Here's how the part is built. I have some questions about the finished solid (model axes, mm). A direction names the side the tool comes from. Give positions to 0.01 mm unless a question says otherwise; leave off trailing zeros. Loops run counter-clockwise (first coordinate to the right, second up) from the corner with the lowest first, then second, coordinate; pieces in that order, holes last. Notation, with made-up numbers: (67, -14) - (110, -14) arc R28 ccw to (110, 19) - close; hole circle Ø4 at (8, 17). An arc over 180 degrees is marked (long way). Return JSON: item names as keys, results as strings. Group by question number.
(1) I need wall thicknesses on probe 1 along Y at (x, z) = (34.5, -22); probe 2 along X at (y, z) = (1, 29.5); probe 3 along X at (y, z) = (7, -34). Which ranges of each line are inside material? Lowest first, please. Write a range as [from, to].
(2) If we section it at A-A (x = 26): Please give me the cut outline in (y, z).
(3) If we mould it in two halves opening along Z, with no side actions, what happens to faces 1 (the flat face through (37, 7.493, 31)), 2 (the cylindrical face through (-92.62, -0.38, 51.75)), 3 (the flat face through (37.2, 6.2, -24.3)), 4 (the flat face through (37.2, 7.239, 27.5))? For each: released by +Z, released by -Z, zero draft, split by the parting line, or undercut.
(4) On a 3-axis mill with a long thin cutter (end or side, diameter ignored), from which of +Z, -Z, +X, -X, +Y, -Y can I reach the whole of each face in a straight line? I mean faces 5 (the flat face through (-19.051, 6.303, 34.262)), 6 (the flat face through (-81.539, 3, -2)), 7 (the flat face through (53, 3, -52.031)). Say none if no direction works.
(5) For P1, Ø3, axis at y = 4.5, z = 35, coming from the -X side; P2, Ø2, axis at x = -68, z = -18.5, coming from the +Y side; P3, Ø2, axis at x = -37.5, y = 4, coming from the -Z side; P4, Ø1.2, axis at y = 6.5, z = 26.5, coming from the -X side, each with a flat end and sliding along its axis, tell me the tip position at first contact or that it passes through.
(6) If we section it at C-C (x = -13): Please give me the cut outline in (y, z).
(7) If we section it at B-B (z = 2.5): Please give me the cut outline in (x, y).
```python
from build123d import *

# Parameters (mm, degrees)
F1_DEPTH   = 0.762
F2_W       = 166.2938
F2_H       = 100.7999
F3_DEPTH   = 5.08
F4_W       = 14.478
F4_H       = 7.874
F4_R       = 1.27
F4_W_2     = 7.874
F4_H_2     = 14.478
F5_DEPTH   = 2.413
F6_SIZE2   = 3.80999
F6_SIZE    = 2.41299
F6_2_SIZE2 = 3.80999
F6_2_SIZE  = 2.41299
F6_3_SIZE2 = 3.80999
F6_3_SIZE  = 2.41299
F6_4_SIZE2 = 3.80999
F6_4_SIZE  = 2.41299
F6_5_SIZE2 = 3.80999
F6_5_SIZE  = 2.41299
F6_6_SIZE2 = 3.80999
F6_6_SIZE  = 2.41299
F6_7_SIZE2 = 3.80999
F6_7_SIZE  = 2.41299
F6_8_SIZE2 = 3.80999
F6_8_SIZE  = 2.41299
F6_9_SIZE2 = 3.80999
F6_9_SIZE  = 2.41299
F7_SIZE2   = 3.80999
F7_SIZE    = 2.41299
F7_2_SIZE2 = 3.80999
F7_2_SIZE  = 2.41299
F7_3_SIZE2 = 3.80999
F7_3_SIZE  = 2.41299
F7_4_SIZE2 = 3.80999
F7_4_SIZE  = 2.41299
F7_5_SIZE2 = 3.80999
F7_5_SIZE  = 2.41299
F7_6_SIZE2 = 3.80999
F7_6_SIZE  = 2.41299
F7_7_SIZE2 = 3.80999
F7_7_SIZE  = 2.41299
F9_DEPTH   = 73.533
F11_DEPTH  = 64.2493
F12_W      = 40.005
F12_H      = 5.08
F13_DEPTH  = 3.34264


# Not quite as in the source:
# - a fillet or chamfer is up to 0.001 mm smaller than in the source, because OpenCascade refuses the exact size


with BuildPart() as f1:
    # F0 (on Front) → F1 (new body)
    with BuildSketch(Plane.XZ):
        with BuildLine():
            ThreePointArc((96.43872, 42.67327), (92.7189761211, 51.6535261211), (83.73872, 55.37327))
            Line((83.73872, 55.37327), (-83.73872, 55.37327))
            ThreePointArc((-83.73872, 55.37327), (-92.7189761211, 51.6535261211), (-96.43872, 42.67327))
            Line((-96.43872, 42.67327), (-96.43872, -42.67327))
            ThreePointArc((-96.43872, -42.67327), (-92.7189761211, -51.6535261211), (-83.73872, -55.37327))
            Line((-83.73872, -55.37327), (83.73872, -55.37327))
            ThreePointArc((83.73872, -55.37327), (92.7189761211, -51.6535261211), (96.43872, -42.67327))
            Line((96.43872, -42.67327), (96.43872, 42.67327))
        make_face()
    extrude(amount=F1_DEPTH)

    # F2 (on face) → F3 (join)
    with BuildSketch(Plane(origin=(0, 0, 0), x_dir=(-1, 0, 0), z_dir=(0, 1, 0))):
        with Locations((-1.60782, -1.63068)):
            Rectangle(F2_W, F2_H)
    extrude(amount=F3_DEPTH)

    # F4 (on face) → F5 (join)
    with BuildSketch(Plane(origin=(0, 5.08, 0), x_dir=(-1, 0, 0), z_dir=(0, 1, 0))):
        with Locations((-63.98768, 33.78327)):
            Rectangle(F4_W, F4_H)
        with Locations((-63.98768, 33.78327)):
            Circle(F4_R, mode=Mode.SUBTRACT)
        with Locations((-63.98768, -31.87573)):
            Rectangle(F4_W, F4_H)
        with Locations((-63.98768, -31.87573)):
            Circle(F4_R, mode=Mode.SUBTRACT)
        with Locations((62.22492, 33.78327)):
            Rectangle(F4_W, F4_H)
        with Locations((62.22492, 33.78327)):
            Circle(F4_R, mode=Mode.SUBTRACT)
        with Locations((62.22492, -31.87573)):
            Rectangle(F4_W, F4_H)
        with Locations((62.22492, -31.87573)):
            Circle(F4_R, mode=Mode.SUBTRACT)
        with Locations((-37.26942, 28.95473)):
            Rectangle(F4_W_2, F4_H_2)
        with Locations((-37.26942, 28.95473)):
            Circle(F4_R, mode=Mode.SUBTRACT)
        with Locations((19.10588, 28.95473)):
            Rectangle(F4_W_2, F4_H_2)
        with Locations((19.10588, 28.95473)):
            Circle(F4_R, mode=Mode.SUBTRACT)
        with Locations((-37.26942, -19.30527)):
            Rectangle(F4_W_2, F4_H_2)
        with Locations((-37.26942, -19.30527)):
            Circle(F4_R, mode=Mode.SUBTRACT)
        with Locations((19.10588, -19.30527)):
            Rectangle(F4_W_2, F4_H_2)
        with Locations((19.10588, -19.30527)):
            Circle(F4_R, mode=Mode.SUBTRACT)
    extrude(amount=F5_DEPTH)

    # F6 (size 2.413 and 3.81 in the source; OpenCascade refuses exactly that, so slightly less here)
    f6_edges = [f1.edges().sort_by_distance(p)[0] for p in [
        (56.74868, 7.493, 33.78327),
    ]]
    f6_side = f1.faces().sort_by_distance((56.74868, 6.2865, 33.78327))[0]
    chamfer(f6_edges, length=F6_SIZE, length2=F6_SIZE2, reference=f6_side)

    # F6#2 (size 2.413 and 3.81 in the source; OpenCascade refuses exactly that, so slightly less here)
    f6_2_edges = [f1.edges().sort_by_distance(p)[0] for p in [
        (71.22668, 7.493, 33.78327),
    ]]
    f6_2_side = f1.faces().sort_by_distance((71.22668, 6.2865, 33.78327))[0]
    chamfer(f6_2_edges, length=F6_2_SIZE, length2=F6_2_SIZE2, reference=f6_2_side)

    # F6#3 (size 2.413 and 3.81 in the source; OpenCascade refuses exactly that, so slightly less here)
    f6_3_edges = [f1.edges().sort_by_distance(p)[0] for p in [
        (56.74868, 7.493, -31.87573),
    ]]
    f6_3_side = f1.faces().sort_by_distance((56.74868, 6.2865, -31.87573))[0]
    chamfer(f6_3_edges, length=F6_3_SIZE, length2=F6_3_SIZE2, reference=f6_3_side)

    # F6#4 (size 2.413 and 3.81 in the source; OpenCascade refuses exactly that, so slightly less here)
    f6_4_edges = [f1.edges().sort_by_distance(p)[0] for p in [
        (37.26942, 7.493, -26.54427),
    ]]
    f6_4_side = f1.faces().sort_by_distance((37.26942, 6.2865, -26.54427))[0]
    chamfer(f6_4_edges, length=F6_4_SIZE, length2=F6_4_SIZE2, reference=f6_4_side)

    # F6#5 (size 2.413 and 3.81 in the source; OpenCascade refuses exactly that, so slightly less here)
    f6_5_edges = [f1.edges().sort_by_distance(p)[0] for p in [
        (37.26942, 7.493, 21.71573),
    ]]
    f6_5_side = f1.faces().sort_by_distance((37.26942, 6.2865, 21.71573))[0]
    chamfer(f6_5_edges, length=F6_5_SIZE, length2=F6_5_SIZE2, reference=f6_5_side)

    # F6#6 (size 2.413 and 3.81 in the source; OpenCascade refuses exactly that, so slightly less here)
    f6_6_edges = [f1.edges().sort_by_distance(p)[0] for p in [
        (-19.10588, 7.493, -26.54427),
    ]]
    f6_6_side = f1.faces().sort_by_distance((-19.10588, 6.2865, -26.54427))[0]
    chamfer(f6_6_edges, length=F6_6_SIZE, length2=F6_6_SIZE2, reference=f6_6_side)

    # F6#7 (size 2.413 and 3.81 in the source; OpenCascade refuses exactly that, so slightly less here)
    f6_7_edges = [f1.edges().sort_by_distance(p)[0] for p in [
        (-19.10588, 7.493, 21.71573),
    ]]
    f6_7_side = f1.faces().sort_by_distance((-19.10588, 6.2865, 21.71573))[0]
    chamfer(f6_7_edges, length=F6_7_SIZE, length2=F6_7_SIZE2, reference=f6_7_side)

    # F6#8 (size 2.413 and 3.81 in the source; OpenCascade refuses exactly that, so slightly less here)
    f6_8_edges = [f1.edges().sort_by_distance(p)[0] for p in [
        (-69.46392, 7.493, 33.78327),
    ]]
    f6_8_side = f1.faces().sort_by_distance((-69.46392, 6.2865, 33.78327))[0]
    chamfer(f6_8_edges, length=F6_8_SIZE, length2=F6_8_SIZE2, reference=f6_8_side)

    # F6#9 (size 2.413 and 3.81 in the source; OpenCascade refuses exactly that, so slightly less here)
    f6_9_edges = [f1.edges().sort_by_distance(p)[0] for p in [
        (-69.46392, 7.493, -31.87573),
    ]]
    f6_9_side = f1.faces().sort_by_distance((-69.46392, 6.2865, -31.87573))[0]
    chamfer(f6_9_edges, length=F6_9_SIZE, length2=F6_9_SIZE2, reference=f6_9_side)

    # F7 (size 2.413 and 3.81 in the source; OpenCascade refuses exactly that, so slightly less here)
    f7_edges = [f1.edges().sort_by_distance(p)[0] for p in [
        (37.26942, 7.493, 36.19373),
    ]]
    f7_side = f1.faces().sort_by_distance((37.26942, 6.2865, 36.19373))[0]
    chamfer(f7_edges, length=F7_SIZE, length2=F7_SIZE2, reference=f7_side)

    # F7#2 (size 2.413 and 3.81 in the source; OpenCascade refuses exactly that, so slightly less here)
    f7_2_edges = [f1.edges().sort_by_distance(p)[0] for p in [
        (71.22668, 7.493, -31.87573),
    ]]
    f7_2_side = f1.faces().sort_by_distance((71.22668, 6.2865, -31.87573))[0]
    chamfer(f7_2_edges, length=F7_2_SIZE, length2=F7_2_SIZE2, reference=f7_2_side)

    # F7#3 (size 2.413 and 3.81 in the source; OpenCascade refuses exactly that, so slightly less here)
    f7_3_edges = [f1.edges().sort_by_distance(p)[0] for p in [
        (37.26942, 7.493, -12.06627),
    ]]
    f7_3_side = f1.faces().sort_by_distance((37.26942, 6.2865, -12.06627))[0]
    chamfer(f7_3_edges, length=F7_3_SIZE, length2=F7_3_SIZE2, reference=f7_3_side)

    # F7#4 (size 2.413 and 3.81 in the source; OpenCascade refuses exactly that, so slightly less here)
    f7_4_edges = [f1.edges().sort_by_distance(p)[0] for p in [
        (-19.10588, 7.493, -12.06627),
    ]]
    f7_4_side = f1.faces().sort_by_distance((-19.10588, 6.2865, -12.06627))[0]
    chamfer(f7_4_edges, length=F7_4_SIZE, length2=F7_4_SIZE2, reference=f7_4_side)

    # F7#5 (size 2.413 and 3.81 in the source; OpenCascade refuses exactly that, so slightly less here)
    f7_5_edges = [f1.edges().sort_by_distance(p)[0] for p in [
        (-19.10588, 7.493, 36.19373),
    ]]
    f7_5_side = f1.faces().sort_by_distance((-19.10588, 6.2865, 36.19373))[0]
    chamfer(f7_5_edges, length=F7_5_SIZE, length2=F7_5_SIZE2, reference=f7_5_side)

    # F7#6 (size 2.413 and 3.81 in the source; OpenCascade refuses exactly that, so slightly less here)
    f7_6_edges = [f1.edges().sort_by_distance(p)[0] for p in [
        (-54.98592, 7.493, 33.78327),
    ]]
    f7_6_side = f1.faces().sort_by_distance((-54.98592, 6.2865, 33.78327))[0]
    chamfer(f7_6_edges, length=F7_6_SIZE, length2=F7_6_SIZE2, reference=f7_6_side)

    # F7#7 (size 2.413 and 3.81 in the source; OpenCascade refuses exactly that, so slightly less here)
    f7_7_edges = [f1.edges().sort_by_distance(p)[0] for p in [
        (-54.98592, 7.493, -31.87573),
    ]]
    f7_7_side = f1.faces().sort_by_distance((-54.98592, 6.2865, -31.87573))[0]
    chamfer(f7_7_edges, length=F7_7_SIZE, length2=F7_7_SIZE2, reference=f7_7_side)

    # F8 (on face) → F9 (cut, through all)
    with BuildSketch(Plane.XY.offset(37.72027)):
        Polygon((-65.5802524895, 7.239), (-68.9891998579, 5.08), (-55.4606401421, 5.08), (-58.8695875105, 7.239), align=None)
        Polygon((60.6323475105, 7.239), (57.2234001421, 5.08), (70.7519598579, 5.08), (67.3430124895, 7.239), align=None)
    extrude(amount=-F9_DEPTH, mode=Mode.SUBTRACT)

    # F10 (on face) → F11 (cut, through all)
    with BuildSketch(Plane(origin=(-23.04288, 0, 0), x_dir=(0, -1, 0), z_dir=(-1, 0, 0))):
        Polygon((-7.239, -22.6606024895), (-5.08, -26.0695498579), (-5.08, -12.5409901421), (-7.239, -15.9499375105), align=None)
        Polygon((-7.239, 25.5993975105), (-5.08, 22.1904501421), (-5.08, 35.7190098579), (-7.239, 32.3100624895), align=None)
    extrude(amount=-F11_DEPTH, mode=Mode.SUBTRACT)

    # F12 (on face) → F13 (join, through all)
    with BuildSketch(Plane(origin=(0, 0, -52.03063), x_dir=(1, 0, 0), z_dir=(0, 0, -1))):
        with Locations((-0.06858, -2.54)):
            Rectangle(F12_W, F12_H)
    extrude(amount=F13_DEPTH)


solid = f1.part
```
Values:
{
 "1": {"probe 1": "[-0.76, 5.08], [7.24, 7.49]", "probe 2": "[-81.54, 84.75]", "probe 3": "[-66.43, -65.96], [-58.49, -58.02], [59.78, 60.25], [67.72, 68.2]"},
 "2": {"outline": "(-0.76, -55.37) - (0, -55.37) - (0, -52.03) - (5.08, -52.03) - (5.08, 48.77) - (0, 48.77) - (0, 55.37) - (-0.76, 55.37) - close"},
 "3": {"face 1": "zero draft", "face 2": "released by +Z", "face 3": "undercut", "face 4": "undercut"},
 "4": {"face 5": "+Z, +Y", "face 6": "+Z, -Z, -X, +Y", "face 7": "-Z, +X, +Y"},
 "5": {"P1": "x = -81.54", "P2": "y = 5.08", "P3": "z = -52.03", "P4": "through"},
 "6": {"outline": "(-0.76, -55.37) - (5.08, -55.37) - (5.08, 48.77) - (0, 48.77) - (0, 55.37) - (-0.76, 55.37) - close"},
 "7": {"outline": "(-96.44, -0.76) - (96.44, -0.76) - (96.44, 0) - (84.75, 0) - (84.75, 5.08) - (-81.54, 5.08) - (-81.54, 0) - (-96.44, 0) - close"}
}
